For this review, take the finished solid that the model builds, in its own axes (mm). Round coordinates to 2 decimals unless told otherwise and drop trailing zeros. Write each loop counter-clockwise with the first axis right and the second up, starting at its lowest first coordinate (ties: lowest second). Pieces come first, ordered by that corner, then holes. Notation, with made-up numbers: (20.25, 5.25) -> (49.25, 5.25) arc R17 ccw to (49.25, 12.25) -> close; hole circle Ø8 at (57, 26). An arc over 180 degrees is marked (long way). Write each question's results on one line, items separated by ' | '. Start each with the question number.
Item 1: Add section B-B (y = 0.8). State the section outline as (x, z) points, plus the area to 3 significant figures.
Item 2: To check wall thickness, follow line 1 along Z through (x, y) = (-35, 0.8); line 2 along Z through (x, y) = (20, 2.15); line 3 along Z through (x, y) = (-36.5, 1.45). State the ranges of each line that lie inside material, in increasing order.
Item 3: Add section A-A (x = 20). State the section outline as (y, z) points (3 decimals).
Item 4: Add section D-D (x = -12). State the section outline as (y, z) points (3 decimals), plus the area to 3 significant figures.
Item 5: Clearance check with a flat-ended pin moving along its axis: pin 1 (1 mm diameter, centred on x = -19.5, y = 1, fed in from -Z). State where the tip first meets the part, or that it passes through.
Item 6: Add section C-C (z = -58.5). State the section outline as (x, y) points (3 decimals).
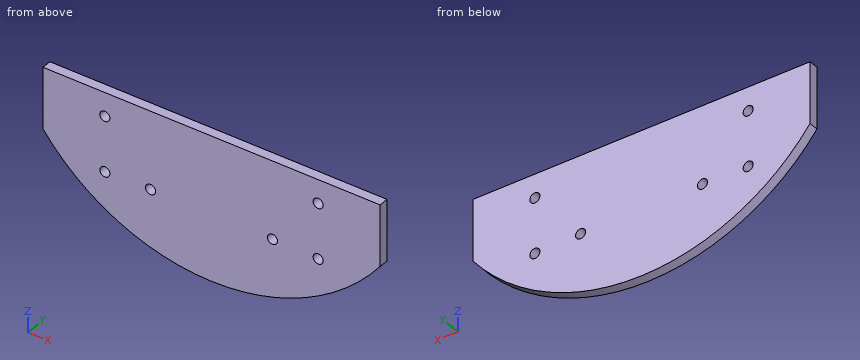
from build123d import *

# Parameters (mm, degrees)
SKETCH1_R           = 1.65
BOSS_EXTRUDE2_DEPTH = 3.175


with BuildPart() as part:
    # Sketch1 → Boss-Extrude2 (new body)
    with BuildSketch(Plane(origin=(0, 0, 0), x_dir=(1, 0, 0), z_dir=(0, 1, 0))):
        with BuildLine():
            Line((-55.306734792, 42.908799641), (-55.306734792, 22.908799641))
            Line((-55.306734792, 22.908799641), (55.306734792, 22.908799641))
            Line((55.306734792, 22.908799641), (55.306734792, 42.908799641))
            ThreePointArc((55.306734792, 42.908799641), (0, 70), (-55.306734792, 42.908799641))
        make_face()
        with Locations((35, 48.621778265)):
            Circle(SKETCH1_R, mode=Mode.SUBTRACT)
        with Locations((35, 30.621778265)):
            Circle(SKETCH1_R, mode=Mode.SUBTRACT)
        with Locations((-35, 30.621778265)):
            Circle(SKETCH1_R, mode=Mode.SUBTRACT)
        with Locations((-35, 48.621778265)):
            Circle(SKETCH1_R, mode=Mode.SUBTRACT)
        with Locations((20, 48.284271247)):
            Circle(SKETCH1_R, mode=Mode.SUBTRACT)
        with Locations((-20, 48.284271247)):
            Circle(SKETCH1_R, mode=Mode.SUBTRACT)
    extrude(amount=BOSS_EXTRUDE2_DEPTH)


solid = part.part
Responses:
1) outline: (-55.31, -42.91) arc R70 ccw to (55.31, -42.91) -> (55.31, -22.91) -> (-55.31, -22.91) -> close; hole circle Ø3.3 at (-35, -48.62); hole circle Ø3.3 at (-35, -30.62); hole circle Ø3.3 at (-20, -48.28); hole circle Ø3.3 at (20, -48.28); hole circle Ø3.3 at (35, -48.62); hole circle Ø3.3 at (35, -30.62) | area: 4,250 mm^2
2) line 1: z = -60.62 to -50.27, -46.97 to -32.27, -28.97 to -22.91 | line 2: z = -67.08 to -49.93, -46.63 to -22.91 | line 3: z = -59.73 to -49.31, -47.93 to -31.31, -29.93 to -22.91
3) outline: (0, -67.082) -> (3.175, -67.082) -> (3.175, -49.934) -> (0, -49.934) -> close; (0, -46.634) -> (3.175, -46.634) -> (3.175, -22.909) -> (0, -22.909) -> close
4) outline: (0, -68.964) -> (3.175, -68.964) -> (3.175, -22.909) -> (0, -22.909) -> close | area: 146 mm^2
5) pin 1: stops at z = -67.37
6) outline: (-38.442, 0) -> (38.442, 0) -> (38.442, 3.175) -> (-38.442, 3.175) -> close
